from build123d import *

# Parameters (mm, degrees)
F1_DEPTH = 132.08
F3_DEPTH = 254.001
F5_DEPTH = 254.001


with BuildPart() as f1:
    # F0 (on Top) → F1 (new body)
    with BuildSketch(Plane.XY):
        Polygon((-127, 76.2), (-127, -76.2), (127, -76.2), (127, 76.2), (88.9, 114.3), (-88.9, 114.3), align=None)
    extrude(amount=F1_DEPTH)

    # F2 (on face) → F3 (cut, through all)
    with BuildSketch(Plane.YZ.offset(127)):
        Polygon((-76.2, 132.08), (-76.2, 0), (-40.809271, 132.08), align=None)
    extrude(amount=-F3_DEPTH, mode=Mode.SUBTRACT)

    # F4 (on face) → F5 (cut, through all)
    with BuildSketch(Plane.YZ.offset(127)):
        Polygon((12.7, 132.08), (-76.2, 132.08), (-76.2, 80.753561), align=None)
    extrude(amount=-F5_DEPTH, mode=Mode.SUBTRACT)


solid = f1.part
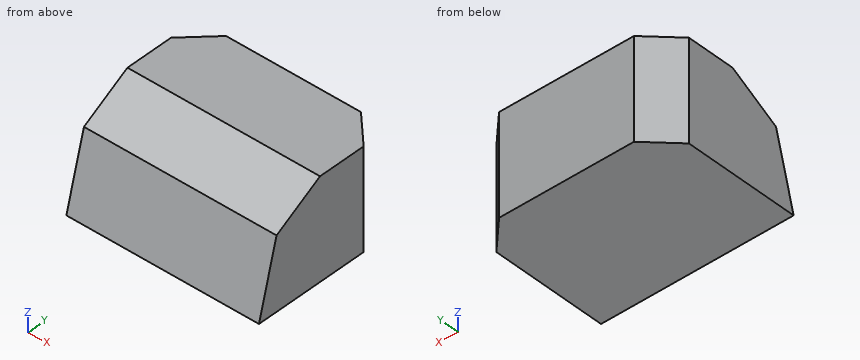
Could you check a few things on this model? Use its own coordinates, in mm. Round coordinates to 2 decimals unless told otherwise and drop trailing zeros. Order: outer loops, then holes, each group sorted by start corner. A loop starts at its lowest first (then second) coordinate and runs counter-clockwise, first axis right, second up.
Q1. Imagine slicing it at D-D, the plane x = 103. List the corners of the cut face in (y, z) for me, then the cut area to 3 significant figures.
Geometry says:
outline: (-76.2, 0) - (100.2, 0) - (100.2, 132.08) - (12.7, 132.08) - (-50.6, 95.53) - close
area: 20,000 mm2
Q2. Please list where these lines run through material, in increasing order: probe 1 along Z at (x, y) = (43, -40.5); probe 2 along X at (y, z) = (91.5, 52.5); probe 3 along X at (y, z) = (77.5, 41).
Geometry says:
probe 1: z = 0 to 101.36
probe 2: x = -111.7 to 111.7
probe 3: x = -125.7 to 125.7
Q3. Imagine slicing it at A-A, the plane x = -96.5. List the corners of the cut face in (y, z) for me.
Geometry says:
outline: (-76.2, 0) - (106.7, 0) - (106.7, 132.08) - (12.7, 132.08) - (-50.6, 95.53) - close
Q4. Imagine slicing it at C-C, the plane y = -27.5. List the corners of the cut face in (x, z) for me, then the cut area to 3 significant figures.
Geometry says:
outline: (-127, 0) - (127, 0) - (127, 108.87) - (-127, 108.87) - close
area: 27,700 mm2
Q5. Imagine slicing it at B-B, the plane z = 63.5. List the corners of the cut face in (x, y) for me.
Geometry says:
outline: (-127, -59.19) - (127, -59.19) - (127, 76.2) - (88.9, 114.3) - (-88.9, 114.3) - (-127, 76.2) - close
Q6. I'm going to push flat-ended pins straight in: P1, Ø12, axis at x = 52, y = -50.5, coming from the +Z side; P2, Ø1, axis at x = 31, z = 55.5, coming from the -Y side. Where does each tip first touch, or does it pass through?
Geometry says:
P1: stops at z = 99.06
P2: stops at y = -61.46
